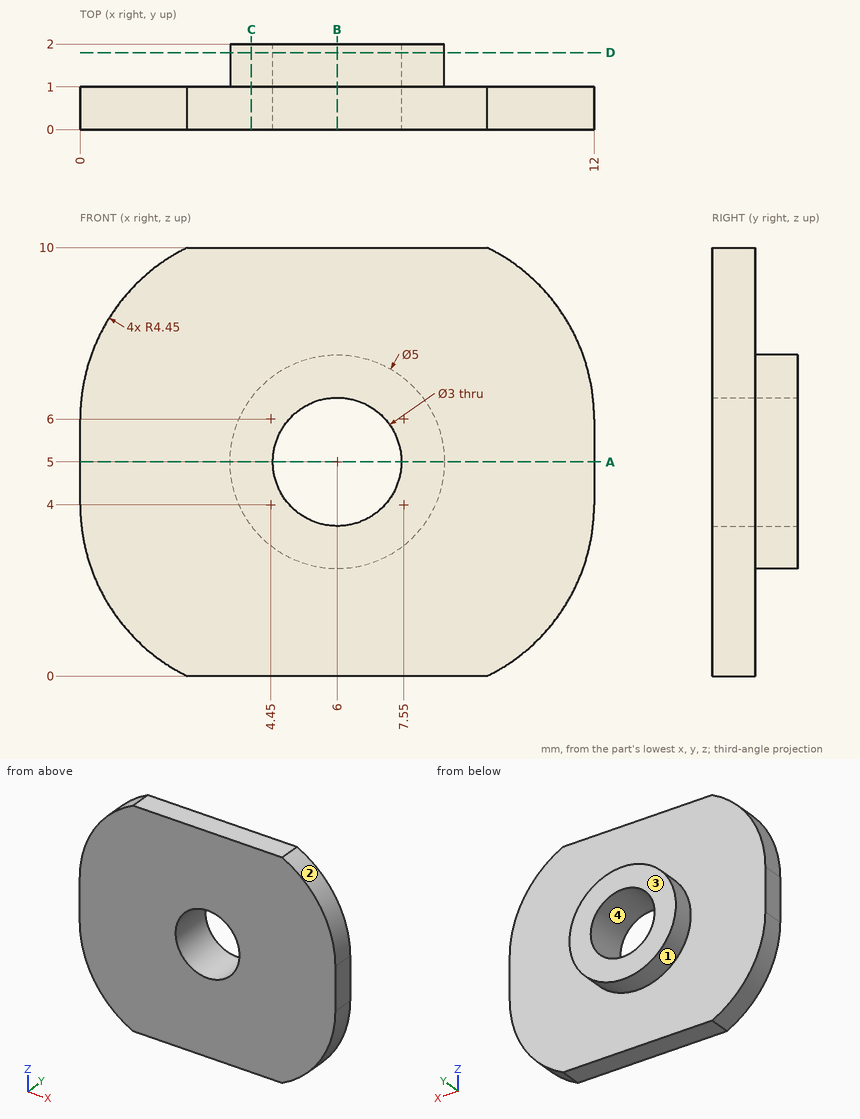
Geometry: see drawing. Coordinates: mm, zero at the bounding-box minimum. Give positions to 0.01 mm unless a question says otherwise; leave off trailing zeros. Order: outer loops, then holes, each group sorted by start corner. A loop starts at its lowest first (then second) coordinate and runs counter-clockwise, first axis right, second up. Notation, with made-up numbers: (-27, 26) -> (18, 26) arc R23 cw to (18, 62) -> close; hole circle Ø5 at (39, 69). An arc over 180 degrees is marked (long way). Write item = value, one per line.
Q1. Pin query (flat end, axial travel): pin 1 (4 mm diameter, centred on x = 6, z = 5, fed in from -Y); pin 2 (1 mm diameter, centred on y = 0.5, z = 2.5, fed in from -X). Return the tip coordinate at first contact, or that it passes through.
Data:
pin_1 = 0
pin_2 = 0.11
Q2. Cut plane B-B, the plane x = 6. Output: boundary loops of the cut face in (y, z).
Data:
outline = (0, 0) -> (1, 0) -> (1, 2.5) -> (2, 2.5) -> (2, 3.5) -> (0, 3.5) -> close; (0, 6.5) -> (2, 6.5) -> (2, 7.5) -> (1, 7.5) -> (1, 10) -> (0, 10) -> close
Q3. Cut plane D-D, the plane y = 1.8. Output: boundary loops of the cut face in (x, z).
Data:
outline = circle Ø5 at (6, 5); hole circle Ø3 at (6, 5)
Q4. Cut plane C-C, the plane x = 4. Output: boundary loops of the cut face in (y, z), and give its area (3 significant figures).
Data:
outline = (0, 0) -> (1, 0) -> (1, 3.5) -> (2, 3.5) -> (2, 6.5) -> (1, 6.5) -> (1, 10) -> (0, 10) -> close
area = 13.0 mm^2
Q5. Cut plane A-A, the plane z = 5. Output: boundary loops of the cut face in (x, y).
Data:
outline = (0, 0) -> (4.5, 0) -> (4.5, 2) -> (3.5, 2) -> (3.5, 1) -> (0, 1) -> close; (7.5, 0) -> (12, 0) -> (12, 1) -> (8.5, 1) -> (8.5, 2) -> (7.5, 2) -> close
Q6. Pull-direction query (X, two-part tool) for the marked faces 1, 2, 3 and 4; classes: released by +X, released by -X, zero draft, split by the parting line, or undercut.
Data:
face_1 = split by the parting line
face_2 = released by +X
face_3 = zero draft
face_4 = undercut
Q7. Material intervals for line 1 (Z direction, x = 6, y = 1.5); line 2 (X direction, y = 0.7, z = 5); line 3 (Z direction, x = 6, y = 0.7), sorted ascending. Write a range as from..to.
Data:
line_1 = 2.5..3.5, 6.5..7.5
line_2 = 0..4.5, 7.5..12
line_3 = 0..3.5, 6.5..10
